Answer from the drawing. Dimensions are ordinates in mm from the lowest x, y and z of the part. Round coordinates to 2 decimals unless told otherwise and drop trailing zeros. Write each loop counter-clockwise with the first axis right and the second up, starting at its lowest first coordinate (ties: lowest second). Pieces come first, ordered by that corner, then holes.
1. Find section B-B (y = 1). Write down the section's boundary in (x, z), and give its area (3 significant figures).
2. Find section A-A (x = 61.5). Write down the section's boundary in (y, z).
3. Flat-ended cylindrical pins translate along their axes: pin 1 Ø4.5 at (x, z) = (5, 34.5) entering from -Y; pin 2 Ø4.5 at (x, z) = (79, 35) entering from -Y; pin 3 Ø10 at (x, z) = (48, 21) entering from -Y. Find the tip coordinate at first contact, or state that the pin passes through.
4. Find section D-D (z = 35). Write down the section's boundary in (x, y), and give its area (3 significant figures).
5. Straight lines are drawn through the part: probe 1 along Z at (x, y) = (79, 0.85); probe 2 along Z at (x, y) = (15, 0.65); probe 3 along X at (y, z) = (3.35, 26.5). For each, find the intervals that lie inside material, in ascending order.
6. Find section C-C (z = 18). Write down the section's boundary in (x, y).
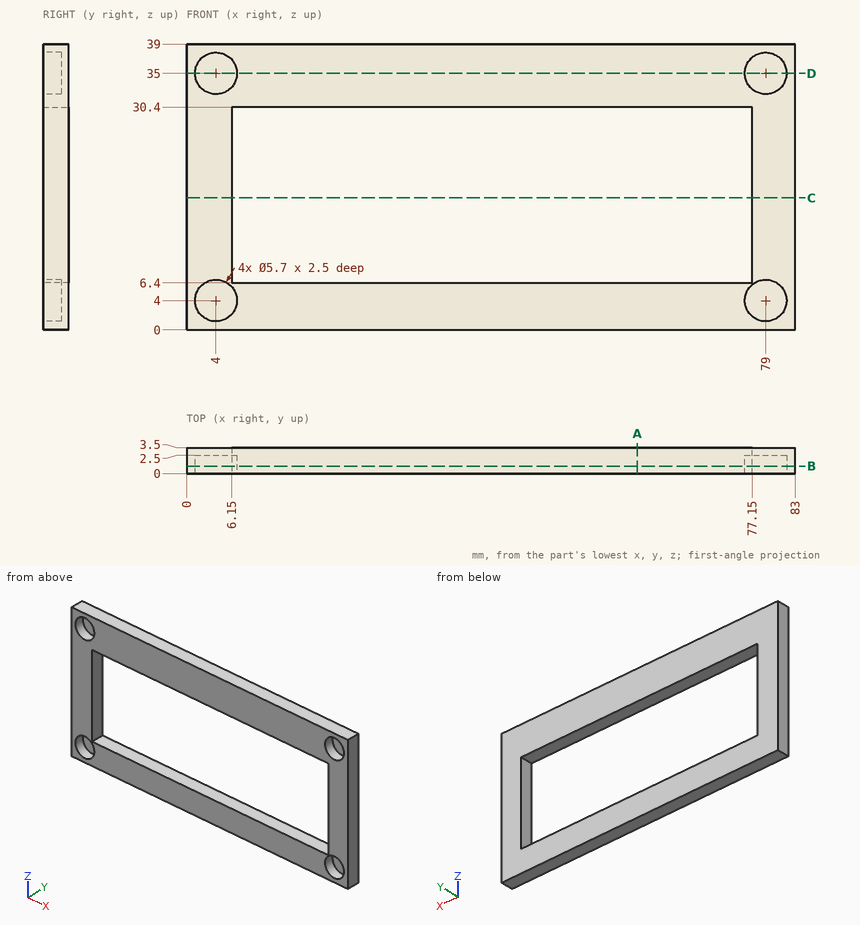
Worked answers:
1. outline: (0, 0) - (83, 0) - (83, 39) - (0, 39) - close; hole circle Ø5.7 at (4, 4); hole circle Ø5.7 at (4, 35); hole (6.15, 6.4) - (77.15, 6.4) - (77.15, 30.4) - (6.15, 30.4) - close; hole circle Ø5.7 at (79, 4); hole circle Ø5.7 at (79, 35)
1. area: 1,430 mm2
2. outline: (0, 0) - (3.5, 0) - (3.5, 6.4) - (0, 6.4) - close; (0, 30.4) - (3.5, 30.4) - (3.5, 39) - (0, 39) - close
3. pin 1: stops at y = 0
3. pin 2: stops at y = 2.5
3. pin 3: passes through
4. outline: (0, 0) - (1.15, 0) - (1.15, 2.5) - (6.85, 2.5) - (6.85, 0) - (76.15, 0) - (76.15, 2.5) - (81.85, 2.5) - (81.85, 0) - (83, 0) - (83, 3.5) - (0, 3.5) - close
4. area: 262 mm2
5. probe 1: z = 0 to 1.15, 6.85 to 32.15, 37.85 to 39
5. probe 2: z = 0 to 6.4, 30.4 to 39
5. probe 3: x = 0 to 6.15, 77.15 to 83
6. outline: (0, 0) - (6.15, 0) - (6.15, 3.5) - (0, 3.5) - close; (77.15, 0) - (83, 0) - (83, 3.5) - (77.15, 3.5) - close
